```python
from build123d import *

# Parameters (mm, degrees)
SKETCH_148_R          = 10
EXTRUDE_195_DEPTH     = 10
CUT_EXTRUDE_296_DEPTH = 5
CHAMFER_1_SIZE        = 2
CHAMFER_1_SIZE2       = 1.154700538


with BuildPart() as part:
    # Sketch 148 → Extrude 195 (new body)
    with BuildSketch(Plane(origin=(0, 0, 0), x_dir=(1, 0, 0), z_dir=(0, 1, 0))):
        with Locations(Location((0, 0, 0), (0, 0, 270))):
            Circle(SKETCH_148_R)
    extrude(amount=EXTRUDE_195_DEPTH)

    # Sketch 234 → Cut-Extrude 296 (cut)
    with BuildSketch(Plane(origin=(0, 0, 0), x_dir=(1, 0, 0), z_dir=(0, 1, 0))):
        with BuildLine():
            Line((-2, -1.5), (2, -1.5))
            ThreePointArc((2, -1.5), (0, 2.5), (-2, -1.5))
        make_face()
    extrude(amount=CUT_EXTRUDE_296_DEPTH, mode=Mode.SUBTRACT)

    # Фаска1
    chamfer_1_edges = [part.edges().sort_by_distance(p)[0] for p in [
        (0, 10, -10),
    ]]
    chamfer_1_side = [part.faces().sort_by_distance(p)[0] for p in [
        (0, 5, -10),
    ]]
    chamfer(chamfer_1_edges, length=CHAMFER_1_SIZE, length2=CHAMFER_1_SIZE2, reference=chamfer_1_side[0])


solid = part.part
```
Verification items for the finished model (mm, model axes). A direction names the side the tool comes from. Give positions to 0.01 mm unless a question says otherwise; leave off trailing zeros. Order: outer loops, then holes, each group sorted by start corner. A loop starts at its lowest first (then second) coordinate and runs counter-clockwise, first axis right, second up. Notation, with made-up numbers: (41, 19.5) - (92, 19.5) arc R6 cw to (92, 24.5) - close; hole circle Ø4 at (3.25, 57.25). An arc over 180 degrees is marked (long way). Answer as CSV lines item,"result". Start each with the question number.
Item 1: Gauge pin test, flat ends, axial feed: pin 1 (8 mm diameter, centred on x = -7.5, z = 7.5, fed in from +Y); pin 2 (1 mm diameter, centred on x = 7, y = 5, fed in from +Z). Record the tip position at first contact, or that the pin passes through.
Item 2: Section check C-C, the plane y = 7.5. Record the boundary of the cut face in (x, z), plus the area to 3 significant figures.
Item 3: Section check A-A, the plane z = 0. Record the boundary of the cut face in (x, y).
Item 4: Section check D-D, the plane y = 1.5. Record the boundary of the cut face in (x, z).
Item 5: Section check B-B, the plane x = 0. Record the boundary of the cut face in (y, z).
Item 6: Mould release check, pull along X, two halves, no side actions. Record for faces 1 (the face through (0, 10, 0)), 2 (the face through (-9.76, 3.94, -2.17)), 3 (the face through (0.1, 2.5, -2.5)): released by +X, released by -X, zero draft, split by the parting line, or undercut.
Item 7: Material ranges on L1, parallel to X at y = 3.4, z = 0; L2, parallel to X at y = 2.5, z = -2; L3, parallel to Z at x = 0.75, y = 1.75, recorded low to high.
Item 8: Access from +Z, -Z, +X, -X, +Y, -Y to the whole of each face (thin tool, end or side, straight path). Record for faces 4 (the face through (0, 2, 1.5)), 5 (the face through (0, 0, 2)).
Filled in:
1,pin 1,"y = 10"
1,pin 2,"z = 7.6"
2,outline,"circle Ø20 at (0, 0)"
2,area,"314 mm^2"
3,outline,"(-10, 0) - (-2.5, 0) - (-2.5, 5) - (2.5, 5) - (2.5, 0) - (10, 0) - (10, 8) - (8.85, 10) - (-8.85, 10) - (-10, 8) - close"
4,outline,"circle Ø20 at (0, 0); hole (-2, 1.5) arc R2.5 ccw (long way) to (2, 1.5) - close"
5,outline,"(0, -10) - (8, -10) - (10, -8.85) - (10, 8.85) - (8, 10) - (0, 10) - (0, 1.5) - (5, 1.5) - (5, -2.5) - (0, -2.5) - close"
6,face 1,"zero draft"
6,face 2,"split by the parting line"
6,face 3,"undercut"
7,L1,"-10 to -2.5, 2.5 to 10"
7,L2,"-9.8 to -1.5, 1.5 to 9.8"
7,L3,"-9.97 to -2.38, 1.5 to 9.97"
8,face 4,"-Y"
8,face 5,"+Z, -Z, +X, -X, -Y"
